Here's how the part is built. I have some questions about the finished solid (model axes, mm). A direction names the side the tool comes from. Round coordinates to 2 decimals unless told otherwise and drop trailing zeros. Order: outer loops, then holes, each group sorted by start corner. A loop starts at its lowest first (then second) coordinate and runs counter-clockwise, first axis right, second up.
```python
from build123d import *

# Parameters (mm, degrees)
F1_DEPTH = 32.5
F3_DEPTH = 2
F4_R     = 8
F5_R     = 2
F7_R     = 4
F8_DEPTH = 5.0144418823


with BuildPart() as f1:
    # F0 (on Right) → F1 (new body)
    with BuildSketch(Plane.YZ):
        Polygon((-32.1455987177, 8), (-32.1455987177, 0), (0, 0), (0, 25), (-5, 25), (-9.0555205563, 2), (-29.1455987177, 5.5424228244), (-29.1455987177, 8), align=None)
    extrude(amount=F1_DEPTH)

    # F2 (on face) → F3 (join)
    with BuildSketch(Plane.YZ.offset(32.5)):
        Polygon((-7.997558672, 8), (-29.1455987177, 8), (-29.1455987177, 5.5424228244), (-9.0555205563, 2), align=None)
    extrude(amount=-F3_DEPTH)

    # F4
    f4_edges = [f1.edges().sort_by_distance(p)[0] for p in [
        (31.5, -7.997559, 8),
        (32.5, -2.5, 25),
    ]]
    fillet(f4_edges, radius=F4_R)

    # F5
    f5_edges = [f1.edges().sort_by_distance(p)[0] for p in [
        (32.5, -32.145599, 4),
    ]]
    fillet(f5_edges, radius=F5_R)

    # F6: F1 across plane


with BuildPart() as f1_1:
    add(f1.part)
    add(f1.part.mirror(Plane.YZ))

    # F7 (on face) → F8 (cut, through all)
    with BuildSketch(Plane(origin=(0, 0, 0), x_dir=(1, 0, 0), z_dir=(0, 0, -1))):
        with Locations((0, 22.1455987177)):
            Circle(F7_R)
    extrude(amount=-F8_DEPTH, mode=Mode.SUBTRACT)


solid = f1_1.part
```
1. I need wall thicknesses on probe 1 along Y at (x, z) = (0, 1.7); probe 2 along X at (y, z) = (-14.5, 7.5); probe 3 along Y at (x, z) = (-26.5, 7). Which ranges of each line are inside material? Lowest first, please.
Evaluation:
probe 1: y = -32.15 to -26.15, -18.15 to 0
probe 2: x = -32.5 to -30.5, 30.5 to 32.5
probe 3: y = -32.15 to -29.15, -8.17 to 0
2. On a 3-axis mill with a long thin cutter (end or side, diameter ignored), from which of +Z, -Z, +X, -X, +Y, -Y can I reach the whole of each face in a straight line? I mean faces 1 (the flat face through (7, -30, 8)), 2 (the flat face through (0.427, -16.728, 3.353)), 3 (the flat face through (0, -2, 25)). Say none if no direction works.
Evaluation:
face 1: +Z, +X, -X, -Y
face 2: +Z
face 3: +Z, +X, -X, +Y, -Y
3. If we section it at B-B, the plane y = -17: Write out the boundary of the cut face in (x, z).
Evaluation:
outline: (-32.5, 0) - (32.5, 0) - (32.5, 8) - (30.5, 8) - (30.5, 3.4) - (-30.5, 3.4) - (-30.5, 8) - (-32.5, 8) - close
4. I'm going to push flat-ended pins straight in: P1, Ø1, axis at x = 5, y = -15.5, coming from the +Z side; P2, Ø5, axis at x = 14.5, y = -23.5, coming from the +Z side; P3, Ø2, axis at x = -11.5, y = -16, coming from the +Z side; P4, Ø10, axis at x = 4.5, y = -26, coming from the -Z side. Where does each tip first touch, or does it pass through?
Evaluation:
P1: stops at z = 3.22
P2: stops at z = 4.99
P3: stops at z = 3.4
P4: stops at z = 0
5. If we section it at C-C, the plane x = -18: Write out the boundary of the cut face in (y, z).
Evaluation:
outline: (-32.15, 0) - (0, 0) - (0, 25) - (-5, 25) - (-9.06, 2) - (-29.15, 5.54) - (-29.15, 8) - (-32.15, 8) - close
6. If we section it at A-A, the plane x = 0: Write out the boundary of the cut face in (y, z).
Evaluation:
outline: (-32.15, 0) - (-26.15, 0) - (-26.15, 5.01) - (-29.15, 5.54) - (-29.15, 8) - (-32.15, 8) - close; (-18.15, 0) - (0, 0) - (0, 25) - (-5, 25) - (-9.06, 2) - (-18.15, 3.6) - close
7. If we mould it in two halves opening along Y, with no side actions, what happens to faces 4 (the cylindrical face through (-31.93, -31.544, 3.944)), 5 (the cylindrical face through (-0.52, -26.11, 1.91)), 6 (the flat face through (0, 0, 12))? For each: released by +Y, released by -Y, zero draft, split by the parting line, or undercut.
Evaluation:
face 4: released by -Y
face 5: undercut
face 6: released by +Y
